Read the model definition and answer for the solid it produces. Units are mm, in the model's axes. Face numbers are marked on the shaded views. A direction names the side the tool comes from. Round coordinates to 2 decimals unless told otherwise and drop trailing zeros. Order: outer loops, then holes, each group sorted by start corner. A loop starts at its lowest first (then second) coordinate and runs counter-clockwise, first axis right, second up.
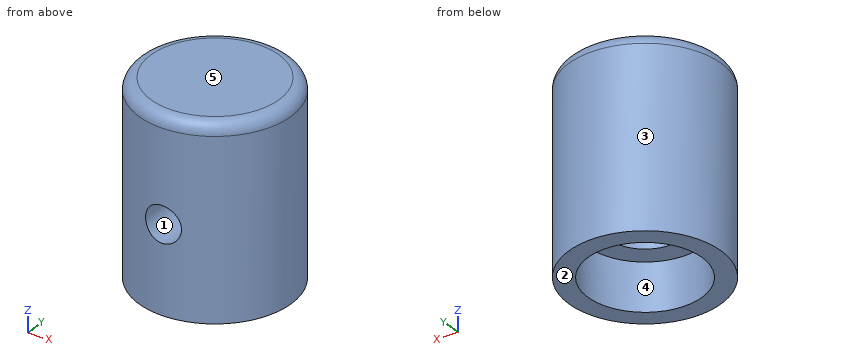
Autodesk Inventor part; units mm, degrees
ref_plane "YZ Plane" through (0, 0, 0) normal (1, 0, 0) x (0, 1, 0)
ref_plane "XZ Plane" through (0, 0, 0) normal (0, 1, 0) x (-1, 0, 0)
ref_plane "XY Plane" through (0, 0, 0) normal (0, 0, 1) x (1, 0, 0)
sketch "Sketch1" plane through (0, 0, 0) normal (0, 0, 1) x (1, 0, 0)
  circle A0 centre (0, 0) radius 6.35
  dimension "d0" = 12.7
extrude "Extrusion1" add sketch "Sketch1" along normal blind 15.875
fillet "Fillet1" radius 1 1 edges at (-6.35, 0, 15.875)
sketch "Sketch2" plane through (0, 0, 0) normal (0, 0, -1) x (-1, 0, 0)
  circle A0 centre (0, 0) radius 4.7625
  dimension "d4" = 9.525
extrude "Extrusion2" cut sketch "Sketch2" against normal blind 3.9878
sketch "Sketch3" plane through (0, 0, 3.9878) normal (0, 0, -1) x (-1, 0, 0)
  circle A0 centre (0, 0) radius 3
  dimension "d7" = 6
extrude "Extrusion3" cut sketch "Sketch3" against normal blind 8.9662
sketch "Sketch4" plane through (0, 0, 0) normal (0, 1, 0) x (-1, 0, 0)
  circle A0 centre (0, 7.239) radius 1.5
  line L0 (6.35, 0) -> (-6.35, 0)
  point P0 (0, 0)
  dimension "d10" = 3
  dimension "d11" = 7.239
extrude "Extrusion4" cut sketch "Sketch4" against normal blind 16.9418
properties part number "Encoder knob"
Q1. For the marked faces 1 and 2, determine the directions among +Z, -Z, +X, -X, +Y, -Y from which every point of the face is accessible in a straight line to the end or side of a thin tool.
Outcome:
face 1: -Y
face 2: -Z, +X, -X, +Y, -Y
Q2. Straight lines are drawn through the part: probe 1 along Z at (x, y) = (2.5, 2) (3 decimals); probe 2 along Y at (x, z) = (0, 3); probe 3 along Z at (x, y) = (1.5, 1.75) (3 decimals). For each, find the intervals that lie inside material, in ascending order.
Outcome:
probe 1: z = 3.988 to 15.875
probe 2: y = -6.35 to -4.76, 4.76 to 6.35
probe 3: z = 12.954 to 15.875
Q3. A cutting plane is placed at D-D, the plane z = 7.5. Give the vertices of the cut face in (x, y), plus the area to 3 significant figures.
Outcome:
outline: (-1.48, -6.18) - (-1.48, -2.61) arc R3 cw (long way) to (1.48, -2.61) - (1.48, -6.18) arc R6.35 ccw (long way) to start
area: 88.3 mm2
Q4. Flat-ended cylindrical pins translate along their axes: pin 1 (5.5 mm diameter, centred on x = 0, y = 0, fed in from -Z); pin 2 (6 mm diameter, centred on x = -1, y = -1.5, fed in from -Z); pin 3 (1 mm diameter, centred on y = 5, z = 2, fed in from +X); pin 4 (1 mm diameter, centred on x = -3.5, y = 1.5, fed in from -Z). Find the tip coordinate at first contact, or state that the pin passes through.
Outcome:
pin 1: stops at z = 12.95
pin 2: stops at z = 0
pin 3: stops at x = 4.48
pin 4: stops at z = 3.99
Q5. For a pull along X with two mould halves and no side action, classify the marked faces 3, 4 and 5 as released by +X, released by -X, zero draft, split by the parting line, or undercut.
Outcome:
face 3: split by the parting line
face 4: undercut
face 5: zero draft
Q6. A cutting plane is placed at C-C, the plane z = 12. Give the vertices of the cut face in (x, y), plus the area to 3 significant figures.
Outcome:
outline: circle Ø12.7 at (0, 0); hole circle Ø6 at (0, 0)
area: 98.4 mm2
